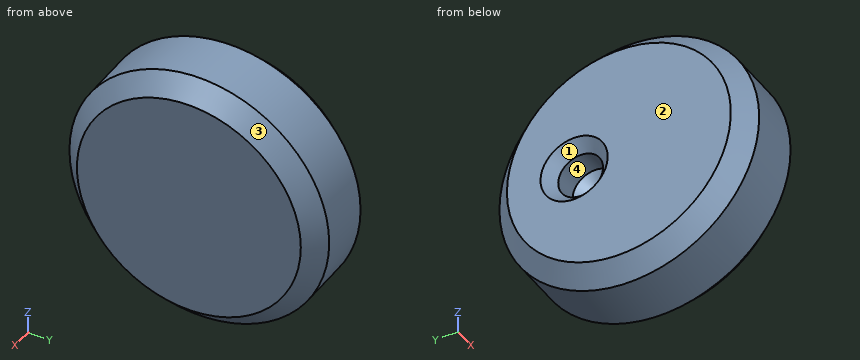
Autodesk Inventor part; units mm, degrees
ref_plane "YZ Plane" through (0, 0, 0) normal (1, 0, 0) x (0, 1, 0)
ref_plane "XZ Plane" through (0, 0, 0) normal (0, 1, 0) x (-1, 0, 0)
ref_plane "XY Plane" through (0, 0, 0) normal (0, 0, 1) x (1, 0, 0)
sketch "Эскиз1" plane through (0, 0, 0) normal (0, 0, 1) x (1, 0, 0)
  line L0 (0, 0) -> (20, 0)
  line L1 (20, 0) -> (20, 25)
  line L2 (16, 29) -> (4, 29)
  line L3 (0, 25) -> (0, 0)
  line L4 (4, 29) -> (0, 25)
  line L5 (16, 29) -> (20, 25)
  point P0 (20, 29)
  point P1 (0, 29)
  dimension "d15" = 20
  dimension "d16" = 29
  dimension "d17" = 4
  dimension "d18" = 4
  dimension "d19" = 4
  dimension "d20" = 4
revolve "Вращение2" add sketch "Эскиз1" angle 360 about axis through (0, 0, 0) along (1, 0, 0)
sketch "Эскиз3" plane through (0, 0, 0) normal (-1, 0, 0) x (0, 0, 1)
  line L0 (0, 0) -> (0, 10) construction
  dimension "d22" = 10
hole "Отверстие2" at (0, 10, 0) direction (1, 0, 0) diameter 10 depth 8 tip angle 118 countersink diameter 15 countersink angle 90
properties part number "711112"
CAD build for the part. Positions are in the model's coordinates, mm. Face numbers are marked on the shaded views. Round coordinates to 2 decimals unless told otherwise and drop trailing zeros. Write each loop counter-clockwise with the first axis right and the second up, starting at its lowest first coordinate (ties: lowest second). Pieces come first, ordered by that corner, then holes. Notation, with made-up numbers: (8, -12.5) - (46, -12.5) arc R19 ccw to (46, -8.5) - close; hole circle Ø1 at (19, -4). An arc over 180 degrees is marked (long way). Write item = value, one per line. Start each with the question number.
Q1. Drop flat-ended pins along their axis: pin 1 (12 mm diameter, centred on x = 9.5, z = -11, fed in from +Y); pin 2 (1.5 mm diameter, centred on x = 7.5, z = 14, fed in from -Y); pin 3 (13 mm diameter, centred on y = 10, z = 0, fed in from -X). Give the stop position or say it passes through.
Q2. Band-saw the part on C-C (x = 13.25). Give the cut face in (y, z).
Q3. Probe L1, parallel to Z at x = 12.25, y = 0.5; L2, parallel to Z at x = 4.9, y = 10; L3, parallel to Y at x = 3.8, z = 0. List the from-to ranges inside material, lowest first. Write a range as from..to.
Q4. Band-saw the part on D-D (x = 9.25). Give the cut face in (y, z).
Q5. Band-saw the part on B-B (x = 1.75). Give the cut face in (y, z).
Q6. Band-saw the part on A-A (y = 0). Give the cut face in (x, z), then the cut area to 3 significant figures.
Q7. Mould opens along Z. For the marked faces 1, 2, 3 and 4 say: pulls with the +Z half, pulls with the -Z half, needs draft (parallel to the pull), parting line crosses it, or undercut.
Answers below:
q1.pin_1 = 28.57
q1.pin_2 = -25.8
q1.pin_3 = 1
q2.outline = circle Ø58 at (0, 0)
q3.L1 = -29..29
q3.L2 = -27.22..-5, 5..27.22
q3.L3 = -28.8..5, 15..28.8
q4.outline = circle Ø58 at (0, 0); hole circle Ø5.84 at (10, 0)
q5.outline = circle Ø53.5 at (0, 0); hole circle Ø11.5 at (10, 0)
q6.outline = (0, -25) - (4, -29) - (16, -29) - (20, -25) - (20, 25) - (16, 29) - (4, 29) - (0, 25) - close
q6.area = 1,130 mm2
q7.face_1 = undercut
q7.face_2 = needs draft
q7.face_3 = parting line crosses it
q7.face_4 = undercut
